from build123d import *

# Parameters (mm, degrees)
F1_DEPTH = 7
F2_SIZE  = 0.5


with BuildPart() as f1:
    # F0 (on Top) → F1 (new body)
    with BuildSketch(Plane.XY):
        Polygon((8.378810594, 18.741624645), (9.614679115, 16.6010375752), (11.146737042, 17.4855716318), (11.146737042, 30.3567148954), (0, 36.7922865272), (-11.146737042, 30.3567148954), (-11.146737042, 17.4855716318), (-9.614679115, 16.6010375752), (-8.378810594, 18.741624645), (-8.675, 18.9126296784), (-8.675, 28.9296568488), (0, 33.938170434), (8.675, 28.9296568488), (8.675, 18.9126296784), align=None)
        with BuildLine():
            Line((-4.0649183257, 13.3968816896), (0, 11.05))
            Line((0, 11.05), (4.0649183257, 13.3968816896))
            ThreePointArc((4.0649183257, 13.3968816896), (2.1359865208, 13.8360963275), (0.1644037795, 13.9990346595))
            Line((0.1644037795, 13.9990346595), (0, 13.9041160931))
            Line((0, 13.9041160931), (-0.1644037795, 13.9990346595))
            ThreePointArc((-0.1644037795, 13.9990346595), (-2.1359865208, 13.8360963275), (-4.0649183257, 13.3968816896))
        make_face()
        with BuildLine():
            ThreePointArc((9.1121955979, 10.6286354433), (10.2458784466, 9.5405437401), (11.2504851637, 8.3322616126))
            Line((11.2504851637, 8.3322616126), (12.8195721533, 11.05))
            Line((12.8195721533, 11.05), (9.614679115, 16.6010375752))
            Line((9.614679115, 16.6010375752), (7.0166029036, 15.1010375752))
            Line((7.0166029036, 15.1010375752), (9.3554705381, 11.05))
            Line((9.3554705381, 11.05), (9.1121955979, 10.6286354433))
        make_face()
        with BuildLine():
            ThreePointArc((7.6044558373, 8.0171535733), (8.6955707884, 6.8183244762), (9.5995515555, 5.4727607232))
            Line((9.5995515555, 5.4727607232), (11.2504851637, 8.3322616126))
            ThreePointArc((11.2504851637, 8.3322616126), (10.2458784466, 9.5405437401), (9.1121955979, 10.6286354433))
            Line((9.1121955979, 10.6286354433), (7.6044558373, 8.0171535733))
        make_face()
        with BuildLine():
            ThreePointArc((0, 11.05), (4.0934675408, 10.2638210961), (7.6044558373, 8.0171535733))
            Line((7.6044558373, 8.0171535733), (9.1121955979, 10.6286354433))
            ThreePointArc((9.1121955979, 10.6286354433), (6.7323754841, 12.2749794436), (4.0649183257, 13.3968816896))
            Line((4.0649183257, 13.3968816896), (0, 11.05))
        make_face()
        with BuildLine():
            Line((-9.1121955979, 10.6286354433), (-7.6044558373, 8.0171535733))
            ThreePointArc((-7.6044558373, 8.0171535733), (-4.0934675408, 10.2638210961), (0, 11.05))
            Line((0, 11.05), (-4.0649183257, 13.3968816896))
            ThreePointArc((-4.0649183257, 13.3968816896), (-6.7323754841, 12.2749794436), (-9.1121955979, 10.6286354433))
        make_face()
        with BuildLine():
            ThreePointArc((9.5995515555, 5.4727607232), (10.6812345889, 2.8308528142), (11.05, 0))
            ThreePointArc((11.05, 0), (-2.8308528142, -10.6812345889), (-9.5995515555, 5.4727607232))
            Line((-9.5995515555, 5.4727607232), (-11.2504851637, 8.3322616126))
            ThreePointArc((-11.2504851637, 8.3322616126), (-4.3870951499, -13.2948635249), (14, 0))
            ThreePointArc((14, 0), (13.2948635249, 4.3870951499), (11.2504851637, 8.3322616126))
            Line((11.2504851637, 8.3322616126), (9.5995515555, 5.4727607232))
        make_face()
        with BuildLine():
            Line((-11.2504851637, 8.3322616126), (-9.5995515555, 5.4727607232))
            ThreePointArc((-9.5995515555, 5.4727607232), (-8.6955707884, 6.8183244762), (-7.6044558373, 8.0171535733))
            Line((-7.6044558373, 8.0171535733), (-9.1121955979, 10.6286354433))
            ThreePointArc((-9.1121955979, 10.6286354433), (-10.2458784466, 9.5405437401), (-11.2504851637, 8.3322616126))
        make_face()
        with BuildLine():
            Line((-12.8195721533, 11.05), (-11.2504851637, 8.3322616126))
            ThreePointArc((-11.2504851637, 8.3322616126), (-10.2458784466, 9.5405437401), (-9.1121955979, 10.6286354433))
            Line((-9.1121955979, 10.6286354433), (-9.3554705381, 11.05))
            Line((-9.3554705381, 11.05), (-7.0166029036, 15.1010375752))
            Line((-7.0166029036, 15.1010375752), (-9.614679115, 16.6010375752))
            Line((-9.614679115, 16.6010375752), (-12.8195721533, 11.05))
        make_face()
        with BuildLine():
            Line((-7.0166029036, 15.1010375752), (-4.0649183257, 13.3968816896))
            ThreePointArc((-4.0649183257, 13.3968816896), (-2.1359865208, 13.8360963275), (-0.1644037795, 13.9990346595))
            Line((-0.1644037795, 13.9990346595), (-5.7807343826, 17.241624645))
            Line((-5.7807343826, 17.241624645), (-7.0166029036, 15.1010375752))
        make_face()
        Polygon((-8.378810594, 18.741624645), (-9.614679115, 16.6010375752), (-7.0166029036, 15.1010375752), (-5.7807343826, 17.241624645), align=None)
        Polygon((7.0166029036, 15.1010375752), (9.614679115, 16.6010375752), (8.378810594, 18.741624645), (5.7807343826, 17.241624645), align=None)
        with BuildLine():
            ThreePointArc((0.1644037795, 13.9990346595), (2.1359865208, 13.8360963275), (4.0649183257, 13.3968816896))
            Line((4.0649183257, 13.3968816896), (7.0166029036, 15.1010375752))
            Line((7.0166029036, 15.1010375752), (5.7807343826, 17.241624645))
            Line((5.7807343826, 17.241624645), (0.1644037795, 13.9990346595))
        make_face()
    extrude(amount=F1_DEPTH)

    # F2
    f2_edges = [f1.edges().sort_by_distance(p)[0] for p in [
        (-11.146737, 23.921143, 7),
        (-5.573369, 33.574501, 7),
        (5.573369, 33.574501, 7),
        (11.146737, 23.921143, 7),
        (10.380708, 17.043305, 7),
        (11.217126, 13.825519, 7),
        (12.035029, 9.691131, 7),
        (0, -14, 7),
        (-12.035029, 9.691131, 7),
        (-11.217126, 13.825519, 7),
        (-10.380708, 17.043305, 7),
        (9.599552, -5.472761, 7),
        (-6.732375, 12.274979, 7),
        (-9.233833, 10.839318, 7),
        (-8.186037, 13.075519, 7),
        (-5.540761, 14.24896, 7),
        (4.3375, 16.408373, 7),
        (-4.3375, 16.408373, 7),
        (-8.675, 23.921143, 7),
        (-4.3375, 31.433914, 7),
        (4.3375, 31.433914, 7),
        (8.675, 23.921143, 7),
        (8.186037, 13.075519, 7),
        (9.233833, 10.839318, 7),
        (6.732375, 12.274979, 7),
        (5.540761, 14.24896, 7),
        (11.217126, 13.825519, 0),
        (10.380708, 17.043305, 0),
        (11.146737, 23.921143, 0),
        (5.573369, 33.574501, 0),
        (-5.573369, 33.574501, 0),
        (-11.146737, 23.921143, 0),
        (-10.380708, 17.043305, 0),
        (-11.217126, 13.825519, 0),
        (-12.035029, 9.691131, 0),
        (0, -14, 0),
        (12.035029, 9.691131, 0),
        (9.599552, -5.472761, 0),
        (-6.732375, 12.274979, 0),
        (-9.233833, 10.839318, 0),
        (-8.186037, 13.075519, 0),
        (-5.540761, 14.24896, 0),
        (4.3375, 16.408373, 0),
        (-4.3375, 16.408373, 0),
        (-8.675, 23.921143, 0),
        (-4.3375, 31.433914, 0),
        (4.3375, 31.433914, 0),
        (8.675, 23.921143, 0),
        (8.186037, 13.075519, 0),
        (9.233833, 10.839318, 0),
        (6.732375, 12.274979, 0),
        (5.540761, 14.24896, 0),
    ]]
    chamfer(f2_edges, length=F2_SIZE)


solid = f1.part
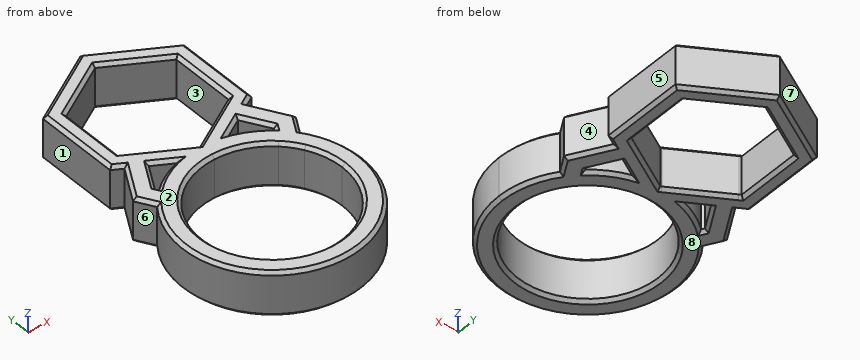
Source: CAD feature listing. Evaluate the final solid. Frame: model axes, mm. Face numbers are marked on the shaded views. A direction names the side the tool comes from. Coordinates: 2 decimals unless noted, no trailing zeros. Order: outer loops, then holes, each group sorted by start corner. A loop starts at its lowest first (then second) coordinate and runs counter-clockwise, first axis right, second up. Notation, with made-up numbers: M 10.5,-10 L 31.5,-10 A15 cw 31.5,15 Z; hole C -24.75,51.25 d1. An arc over 180 degrees is marked long. Write each question's results on one line, items separated by ' | '. Start each with the question number.
Item 1: Set-up query: the marked faces 1, 2, 3, 4 and 5. Return all of +Z, -Z, +X, -X, +Y, -Y with unobstructed straight access to the full face (end or side cutting, diameter ignored); none if empty.
Item 2: Line query: probe 1 along Y at (x, z) = (0, 3.7); probe 2 along Y at (x, z) = (7, 3); probe 3 along X at (y, z) = (20.5, 3.5) (3 decimals). Output: solid intervals per line, ascending.
Item 3: Cut plane C-C (y = 32). Return loops of the section in (x, z), and give its area (3 significant figures).
Item 4: Draft query along Y for the marked faces 6, 7 and 8. Return one class per face: pulls with the +Y half, pulls with the -Y half, needs draft (parallel to the pull), parting line crosses it, or undercut.
Item 5: First-contact query: pin 1 Ø3 at (y, z) = (11.5, 3.5) entering from +X; pin 2 Ø1.5 at (x, z) = (8, 3) entering from +Y; pin 3 Ø3 at (y, z) = (22.5, 3.5) entering from -X. Flat tips, straight axial feed; report the tip coordinate or a pass-through.
Item 6: Cut plane A-A (y = 20). Return loops of the section in (x, z) (3 decimals), and give its area (3 significant figures).
Item 7: Cut plane B-B (z = 2.75). Return loops of the section in (x, y) (3 decimals), and give its area (3 significant figures).
Checked values:
1) face 1: +Z, -Z, -X, +Y | face 2: +Z, +X, -X, +Y, -Y | face 3: +Z, -Z | face 4: +Z, -Z, +X | face 5: +Z, -Z, +X, +Y
2) probe 1: y = -14 to -11.05, 11.05 to 13.9, 33.94 to 36.79 | probe 2: y = -12.12 to -8.55, 8.55 to 12.12, 15.09 to 17.95, 29.9 to 32.75 | probe 3: x = -11.147 to -8.675, 8.675 to 11.147
3) outline: M -8.3,0.5 L -7.3,0 L -4.36,0 L -3.36,0.5 L -3.36,6.5 L -4.36,7 L -7.3,7 L -8.3,6.5 Z; M 3.36,0.5 L 4.36,0 L 7.3,0 L 8.3,0.5 L 8.3,6.5 L 7.3,7 L 4.36,7 L 3.36,6.5 Z | area: 67.2 mm2
4) face 6: undercut | face 7: pulls with the +Y half | face 8: needs draft
5) pin 1: stops at x = 12.82 | pin 2: stops at y = 32.61 | pin 3: stops at x = -11.15
6) outline: M -11.147,0.5 L -10.647,0 L -9.175,0 L -8.675,0.5 L -8.675,6.5 L -9.175,7 L -10.647,7 L -11.147,6.5 Z; M 8.675,0.5 L 9.175,0 L 10.647,0 L 11.147,0.5 L 11.147,6.5 L 10.647,7 L 9.175,7 L 8.675,6.5 Z | area: 33.6 mm2
7) outline: M -12.82,11.05 L -11.25,8.332 A14 ccw long 11.25,8.332 L 12.82,11.05 L 9.615,16.601 L 11.147,17.486 L 11.147,30.357 L 0,36.792 L -11.147,30.357 L -11.147,17.486 L -9.615,16.601 Z; hole C 0,0 d22.1; hole M -9.355,11.05 L -9.112,10.629 A14 cw -4.065,13.397 L -7.017,15.101 Z; hole M -8.675,18.913 L 0,13.904 L 8.675,18.913 L 8.675,28.93 L 0,33.938 L -8.675,28.93 Z; hole M 4.065,13.397 A14 cw 9.112,10.629 L 9.355,11.05 L 7.017,15.101 Z | area: 433 mm2
